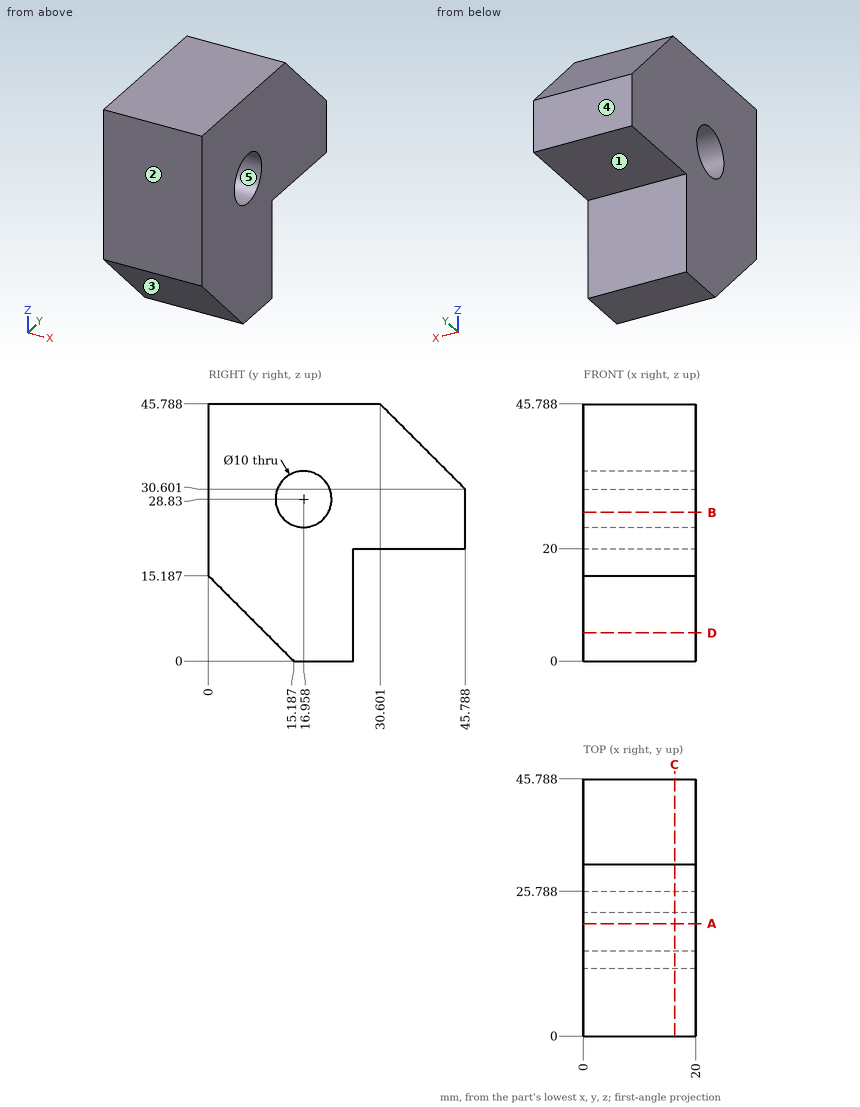
Job drawing, mm, ordinate dimensions from the low corner. One solid piece. A direction names the side the tool comes from. Give positions to 0.01 mm unless a question says otherwise; leave off trailing zeros. Loops run counter-clockwise (first coordinate to the right, second up) from the corner with the lowest first, then second, coordinate; pieces in that order, holes last. Notation, with made-up numbers: M 79.25,64.5 L 108.25,64.5 A18 ccw 108.25,85.5 Z; hole C 4.5,19.5 d5. An arc over 180 degrees is marked long. Put each result on its own line as item: value. Start each with the question number.
1) 3-axis set-ups, long thin cutter, end or side, ignore diameter. For the marked faces 1 and 2: which of +Z, -Z, +X, -X, +Y, -Y reach the whole face in a straight line?
2) Saw through at D-D (z = 5). List the corners of the cut face in (x, y).
3) Pull direction Z, two halves, no side cores. Call the marked faces 3, 4 and 5: +Z half, -Z half, draft (parallel to the pull), parting line (faces both ways), or undercut.
4) Saw through at B-B (z = 26.5). List the corners of the cut face in (x, y).
5) Saw through at C-C (x = 16.25). List the corners of the cut face in (y, z), then the cut area to 3 significant figures.
6) Probe probe 1 along Z at (x, y) = (2.75, 28); probe 2 along Y at (x, z) = (14, 29) (1 decimal); probe 3 along Z at (x, y) = (13.5, 18.5) (1 decimal). List the from-to ranges inside material, lowest first.
7) Saw through at A-A (y = 20). List the corners of the cut face in (x, z).
8) Flat gauge pins, fed straight in: pin 1 (4 mm diameter, centred on x = 4.5, z = 7.5, fed in from +Y); pin 2 (4 mm diameter, centred on y = 23, z = 40.5, fed in from -X); pin 3 (1.5 mm diameter, centred on x = 10.5, z = 11, fed in from -Y); pin 4 (4 mm diameter, centred on x = 17.5, y = 38.5, fed in from -Z). Where does each tip first touch, or does it go through?
Numbers:
1. face 1: -Z, +X, -X, +Y
1. face 2: +Z, -Z, +X, -X, -Y
2. outline: M 0,10.19 L 20,10.19 L 20,25.79 L 0,25.79 Z
3. face 3: -Z half
3. face 4: draft
3. face 5: undercut
4. outline: M 0,0 L 20,0 L 20,12.53 L 0,12.53 Z; M 0,21.38 L 20,21.38 L 20,45.79 L 0,45.79 Z
5. outline: M 0,15.19 L 15.19,0 L 25.79,0 L 25.79,20 L 45.79,20 L 45.79,30.6 L 30.6,45.79 L 0,45.79 Z; hole C 16.96,28.83 d10
5. area: 1,390 mm^2
6. probe 1: 20 to 45.79
6. probe 2: 0 to 12, 22 to 45.8
6. probe 3: 0 to 24.1, 33.6 to 45.8
7. outline: M 0,0 L 20,0 L 20,24.86 L 0,24.86 Z; M 0,32.8 L 20,32.8 L 20,45.79 L 0,45.79 Z
8. pin 1: y = 25.79
8. pin 2: x = 0
8. pin 3: y = 3.44
8. pin 4: z = 20
